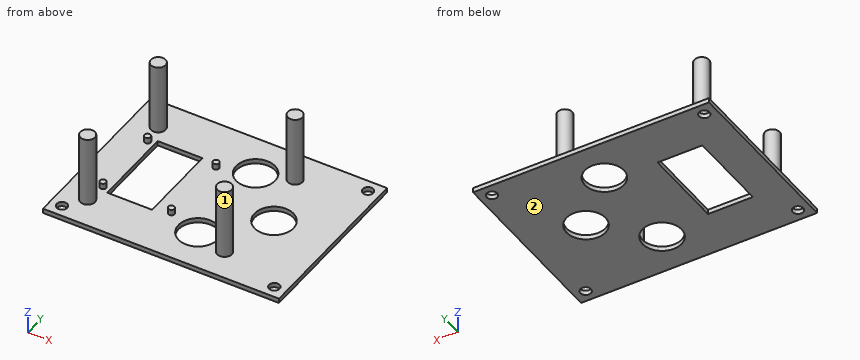
```python
from build123d import *

# Parameters (mm, degrees)
SKETCH_W     = 100
SKETCH_H     = 75
SKETCH_R     = 8.25
SKETCH_R_2   = 2.25
SKETCH_W_2   = 19
SKETCH_H_2   = 35
PAD001_DEPTH = 2
SKETCH008_R  = 1.3
PAD006_DEPTH = 2.5
SKETCH009_R  = 3.1
PAD007_DEPTH = 30


with BuildPart() as part:
    # Sketch → Pad001 (new body)
    with BuildSketch(Plane.XY):
        Rectangle(SKETCH_W, SKETCH_H)
        with Locations((5, 20)):
            Circle(SKETCH_R, mode=Mode.SUBTRACT)
        with Locations((5, -20)):
            Circle(SKETCH_R, mode=Mode.SUBTRACT)
        with Locations((-45, 32.5)):
            Circle(SKETCH_R_2, mode=Mode.SUBTRACT)
        with Locations((-45, -32.5)):
            Circle(SKETCH_R_2, mode=Mode.SUBTRACT)
        with Locations((45, 32.5)):
            Circle(SKETCH_R_2, mode=Mode.SUBTRACT)
        with Locations((45, -32.5)):
            Circle(SKETCH_R_2, mode=Mode.SUBTRACT)
        with Locations((25, 0)):
            Circle(SKETCH_R, mode=Mode.SUBTRACT)
        with Locations((-25.5, 0)):
            Rectangle(SKETCH_W_2, SKETCH_H_2, mode=Mode.SUBTRACT)
    extrude(amount=PAD001_DEPTH)

    # Sketch008 (on Face17 of Pad001) → Pad006 (join)
    with BuildSketch(Plane.XY.offset(2)):
        with Locations((-38, 15.5)):
            Circle(SKETCH008_R)
        with Locations((-9, 15.5)):
            Circle(SKETCH008_R)
        with Locations((-38, -15.5)):
            Circle(SKETCH008_R)
        with Locations((-9, -15.5)):
            Circle(SKETCH008_R)
    extrude(amount=PAD006_DEPTH)

    # Sketch009 (on Face5 of Pad006) → Pad007 (join)
    with BuildSketch(Plane.XY.offset(2)):
        with Locations((19, 24.5)):
            Circle(SKETCH009_R)
        with Locations((-39, 24.5)):
            Circle(SKETCH009_R)
        with Locations((-39, -24.5)):
            Circle(SKETCH009_R)
        with Locations((19, -24.5)):
            Circle(SKETCH009_R)
    extrude(amount=PAD007_DEPTH)


with BuildPart() as part_1:
    # Body placement: moved
    add(part.part.moved(Location((0, 0, -2))))


solid = part_1.part
```
The model under review builds one solid part; all positions refer to its coordinate system, in mm. Face numbers are marked on the shaded views. Give positions to 0.01 mm unless a question says otherwise; leave off trailing zeros. Write each loop counter-clockwise with the first axis right and the second up, starting at its lowest first coordinate (ties: lowest second). Pieces come first, ordered by that corner, then holes. Notation, with made-up numbers: (87, -26.75) - (91, -26.75) arc R30 cw to (91, -0.75) - close; hole circle Ø10 at (74.5, -32.5). An arc over 180 degrees is marked (long way). Answer in a Markdown table with one row per item. Add a question column.
1. We need section A-A on x = 25. Write out the cut boundary in (y, z).
2. Draft analysis for pull direction X (two halves, no side actions). For the marked faces 1 and 2, state which applies: +X half, -X half, draft (parallel to the pull), parting line (faces both ways), or undercut.
3. We need section B-B on y = 32.5. Write out the cut boundary in (x, z).
4. Insertion check: P1, Ø5, axis at x = 19.5, y = 16.5, coming from the +Z side; P2, Ø0.8, axis at x = -37.5, y = -15.5, coming from the +Z side; P3, Ø2, axis at y = -23.5, z = 3, coming from the +X side. Each pin has a flat end and moves straight along its axis. Give the tip position at first contact, or say it passes through.
5. Wall thickness on line 1 along Y through (x, z) = (45, -1); line 2 along Y through (x, z) = (5, -1); line 3 along Z through (x, y) = (19.5, 34): over which ranges is each line inside the solid? List them lowest first. Write a range as [from, to].
6. We need section D-D on x = 45. Write out the cut boundary in (y, z), then the cut area to 3 significant figures.
7. We need section C-C on y = 20. Write out the cut boundary in (x, z), then the cut area to 3 significant figures.
Ans:
| question | item | result |
|---|---|---|
| 1 | outline | (-37.5, -2) - (-8.25, -2) - (-8.25, 0) - (-37.5, 0) - close; (8.25, -2) - (37.5, -2) - (37.5, 0) - (8.25, 0) - close |
| 2 | face 1 | undercut |
| 2 | face 2 | draft |
| 3 | outline | (-50, -2) - (-47.25, -2) - (-47.25, 0) - (-50, 0) - close; (-42.75, -2) - (42.75, -2) - (42.75, 0) - (-42.75, 0) - close; (47.25, -2) - (50, -2) - (50, 0) - (47.25, 0) - close |
| 4 | P1 | stops at z = 0 |
| 4 | P2 | stops at z = 2.5 |
| 4 | P3 | stops at x = 22.1 |
| 5 | line 1 | y = [-37.5, -34.75], [-30.25, 30.25], [34.75, 37.5] |
| 5 | line 2 | y = [-37.5, -28.25], [-11.75, 11.75], [28.25, 37.5] |
| 5 | line 3 | z = [-2, 0] |
| 6 | outline | (-37.5, -2) - (-34.75, -2) - (-34.75, 0) - (-37.5, 0) - close; (-30.25, -2) - (30.25, -2) - (30.25, 0) - (-30.25, 0) - close; (34.75, -2) - (37.5, -2) - (37.5, 0) - (34.75, 0) - close |
| 6 | area | 132 mm^2 |
| 7 | outline | (-50, -2) - (-3.25, -2) - (-3.25, 0) - (-50, 0) - close; (13.25, -2) - (50, -2) - (50, 0) - (13.25, 0) - close |
| 7 | area | 167 mm^2 |
